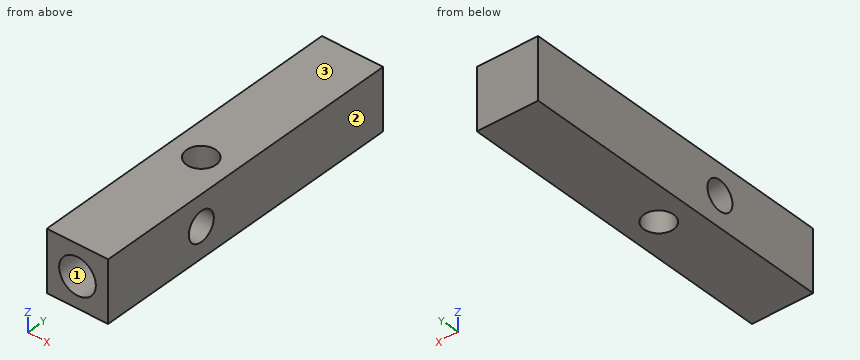
```python
from build123d import *

# Parameters (mm, degrees)
SKETCH_W        = 17
SKETCH_H        = 90
PAD_DEPTH       = 17
SKETCH001_R     = 5.1
POCKET_DEPTH    = 25
SKETCH002_R     = 4.1
POCKET001_DEPTH = 17.001
SKETCH003_R     = 4.1
POCKET002_DEPTH = 17.001


with BuildPart() as part:
    # Sketch → Pad (new body)
    with BuildSketch(Plane.XY):
        with Locations((8.5, 45)):
            Rectangle(SKETCH_W, SKETCH_H)
    extrude(amount=PAD_DEPTH)

    # Sketch001 → Pocket (cut)
    with BuildSketch(Plane.XZ):
        with Locations((8.5, 8.5)):
            Circle(SKETCH001_R)
    extrude(amount=-POCKET_DEPTH, mode=Mode.SUBTRACT)

    # Sketch002 → Pocket001 (cut, through all)
    with BuildSketch(Plane.XY.offset(17)):
        with Locations((8.5, 40.5)):
            Circle(SKETCH002_R)
    extrude(amount=-POCKET001_DEPTH, mode=Mode.SUBTRACT)

    # Sketch003 → Pocket002 (cut, through all)
    with BuildSketch(Plane.YZ.offset(17)):
        with Locations((30.5, 8.5)):
            Circle(SKETCH003_R)
    extrude(amount=-POCKET002_DEPTH, mode=Mode.SUBTRACT)


solid = part.part
```
Could you check a few things on this model? Use its own coordinates, in mm. Face numbers are marked on the shaded views. Give positions to 0.01 mm unless a question says otherwise; leave off trailing zeros. Write each loop counter-clockwise with the first axis right and the second up, starting at its lowest first coordinate (ties: lowest second). Pieces come first, ordered by that corner, then holes. Notation, with made-up numbers: (-4, 20.5) - (47, 20.5) arc R28 cw to (47, 42.5) - close; hole circle Ø6 at (65, -16). An arc over 180 degrees is marked (long way). One line per item, written item: value. Start each with the question number.
Item 1: Please list where these lines run through material, in increasing order: line 1 (Z direction, x = 11, y = 30.5); line 2 (Z direction, x = 8.5, y = 6.75); line 3 (Y direction, x = 7.25, z = 4.75). Write a range as from..to.
Item 2: I'm going to push flat-ended pins straight in: pin 1 (5 mm diameter, centred on x = 8.5, y = 40.5, fed in from +Z); pin 2 (5 mm diameter, centred on x = 8, z = 10, fed in from -Y). Where does each tip first touch, or does it pass through?
Item 3: Imagine slicing it at C-C, the plane y = 30.5. List the corners of the cut face in (x, z) for me.
Item 4: Imagine slicing it at B-B, the plane x = 8.5. List the corners of the cut face in (y, z) for me.
Item 5: If we mould it in two halves opening along Z, with no side actions, what happens to the marked faces 1, 2 and 3? For each: +Z half, -Z half, draft (parallel to the pull), parting line (faces both ways), or undercut.
Item 6: Imagine slicing it at A-A, the plane z = 8.5. List the corners of the cut face in (x, y) for me.
Geometry says:
1. line 1: 0..4.4, 12.6..17
1. line 2: 0..3.4, 13.6..17
1. line 3: 25..28.84, 32.16..36.6, 44.4..90
2. pin 1: through
2. pin 2: y = 25
3. outline: (0, 0) - (17, 0) - (17, 4.4) - (0, 4.4) - close; (0, 12.6) - (17, 12.6) - (17, 17) - (0, 17) - close
4. outline: (0, 0) - (36.4, 0) - (36.4, 17) - (0, 17) - (0, 13.6) - (25, 13.6) - (25, 3.4) - (0, 3.4) - close; (44.6, 0) - (90, 0) - (90, 17) - (44.6, 17) - close; hole circle Ø8.2 at (30.5, 8.5)
5. face 1: undercut
5. face 2: draft
5. face 3: +Z half
6. outline: (0, 0) - (3.4, 0) - (3.4, 25) - (13.6, 25) - (13.6, 0) - (17, 0) - (17, 26.4) - (0, 26.4) - close; (0, 34.6) - (17, 34.6) - (17, 90) - (0, 90) - close; hole circle Ø8.2 at (8.5, 40.5)
